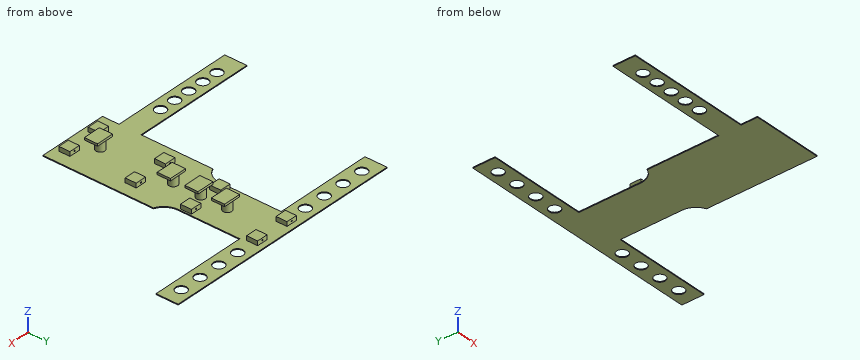
Autodesk Fusion 360 part; units mm, degrees
sketch "Sketch2" plane through (0, 0, 0) normal (0, 0, 1) x (1, 0, 0)
  circle A0 centre (0, 0) radius 11.5
  line L0 (0, 0) -> (0, -11.5)
  line L1 (9.9593, -5.75) -> (-9.9593, -5.75)
  line L2 (9.9593, -5.75) -> (-9.9593, -5.75)
  arc A1 (-9.9593, -5.75) -> (9.9593, -5.75) centre (0, 0) ccw
  dimension "d6" = 23
sketch "Sketch3" plane through (0, 0, 0) normal (0, 0, 1) x (1, 0, 0)
  line L0 (0, -37.5) -> (0, -12.5)
  line L1 (0, -12.5) -> (0, -7.5)
  line L2 (0, -7.5) -> (0, 7.5)
  line L3 (0, 7.5) -> (0, 12.5)
  line L4 (0, 12.5) -> (0, 32.5)
  line L5 (0, 32.5) -> (0, 57.5)
  line L6 (0, 57.5) -> (48, 57.5)
  line L7 (48, 57.5) -> (48, 47.5)
  line L8 (48, 47.5) -> (0, 47.5)
  line L9 (0, 47.5) -> (-48, 47.5)
  line L10 (-48, 57.5) -> (0, 57.5)
  line L11 (0, 32.5) -> (-47.7177, 32.5)
  line L12 (-24, -25) -> (-72, -25)
  line L13 (-72, -25) -> (-72, -20)
  line L14 (-72, -20) -> (-24, -20)
  line L15 (-24, -20) -> (-24, -30)
  line L16 (-24, -30) -> (-72, -30)
  line L17 (-72, -30) -> (-72, -20)
  line L18 (15.8003, -25) -> (15.8003, -28)
  line L19 (-72, -30) -> (-62, -30) construction
  line L20 (-62, -30) -> (-62, -11.1593) construction
  line L21 (-62, -30) -> (-47, -30) construction
  line L22 (-47, -30) -> (-32, -30) construction
  line L23 (-47, -30) -> (-47, -8.6093) construction
  line L24 (-32, -30) -> (-32, -9.4061) construction
  circle A0 centre (-62, -25) radius 2.5
  circle A1 centre (-47, -25) radius 2.5
  circle A2 centre (-32, -25) radius 2.5
  line L25 (-11, 22.5) -> (-11, 25.5)
  line L26 (-11, 19.5) -> (-11, 22.5)
  line L27 (12, 22.5) -> (11, 22.5)
  line L28 (11, 22.5) -> (11, 25.5)
  line L29 (11, 19.5) -> (11, 22.5)
  line L30 (48, 52.5) -> (38, 52.5) construction
  circle A3 centre (-38, 52.5) radius 2.5
  circle A4 centre (38, 52.5) radius 2.5
  line L31 (-38, 52.5) -> (-28, 52.5)
  line L32 (38, 52.5) -> (28, 52.5)
  circle A5 centre (28, 52.5) radius 2.5
  circle A6 centre (-28, 52.5) radius 2.5
  line L33 (-15.8, -12.5) -> (-15.8, 12.5)
  line L34 (11, 25.5) -> (11, 47.5)
  line L35 (-11, 25.5) -> (-11, 47.5)
  line L36 (-15.8, -12.5) -> (-15.8, -37.5)
  line L37 (15.8, 10) -> (15.8003, -22)
  line L38 (-24, -20) -> (-15.8, -20)
  line L39 (-24, -30) -> (-15.8, -30)
  line L40 (-15.8, -37.5) -> (15.8003, -37.5)
  line L41 (15.8003, -22) -> (15.8003, -37.5)
  circle A7 centre (0, -25) radius 2
  line L42 (-2, -25) -> (-3, -25)
  line L43 (-3, -25) -> (-3, -22)
  line L44 (-3, -22) -> (5, -22)
  line L45 (5, -22) -> (5, -28)
  line L46 (5, -28) -> (-3, -28)
  line L47 (-3, -28) -> (-3, -25)
  line L48 (-34.5, -25) -> (-39.5, -25)
  line L49 (-49.5, -25) -> (-54.5, -25)
  circle A8 centre (-39.5, -25) radius 2.5
  circle A9 centre (-54.5, -25) radius 2.5
  line L50 (-15.8, 12.5) -> (15.8, 12.5003)
  line L51 (15.8, 12.5003) -> (15.8, 10)
  arc A10 (-15.8, 12.5) -> (-11, 19.5) centre (-18.5042, 19.5) ccw
  arc A11 (11, 19.5) -> (15.8, 12.5003) centre (18.5037, 19.5) ccw
  circle A12 centre (23, 52.5) radius 2.5 construction
  circle A13 centre (18, 52.5) radius 2.5
  circle A14 centre (-23, 52.5) radius 2.5 construction
  circle A15 centre (-18, 52.5) radius 2.5
  circle A16 centre (43, 52.5) radius 2.5 construction
  circle A17 centre (48, 52.5) radius 2.5
  circle A18 centre (-48, 52.5) radius 2.5
  circle A19 centre (0, 32.5) radius 2
  circle A20 centre (0, 20.5) radius 2
  circle A21 centre (0, 8) radius 2
  line L52 (-2, 8) -> (-3, 8)
  line L53 (-3, 8) -> (-3, 11)
  line L54 (-3, 11) -> (5, 11)
  line L55 (5, 11) -> (5, 5)
  line L56 (5, 5) -> (-3, 5)
  line L57 (-3, 8) -> (-3, 5)
  line L58 (-2, 20.5) -> (-3, 20.5)
  line L59 (-3, 20.5) -> (-3, 23.5)
  line L60 (-3, 23.5) -> (5, 23.5)
  line L61 (5, 23.5) -> (5, 17.5)
  line L62 (5, 17.5) -> (-3, 17.5)
  line L63 (-3, 17.5) -> (-3, 20.5)
  line L64 (-2, 32.5) -> (-3, 32.5)
  line L65 (-3, 32.5) -> (-3, 35.5)
  line L66 (-3, 35.5) -> (5, 35.5)
  line L67 (5, 35.5) -> (5, 29.5)
  line L68 (5, 29.5) -> (-3, 29.5)
  line L69 (-3, 29.5) -> (-3, 32.5)
  line L70 (55.5, 57.5) -> (55.5, 47.5)
  line L71 (48, 47.5) -> (55.5, 47.5)
  line L72 (55.5, 57.5) -> (48, 57.5)
  line L73 (-55.5, 52.5) -> (-55.5, 57.5)
  line L74 (-55.5, 57.5) -> (-48, 57.5)
  line L75 (-48, 47.5) -> (-55.5, 47.5)
  line L76 (-55.5, 47.5) -> (-55.5, 52.5)
  line L77 (15.8003, -37.5) -> (7.8003, -37.5)
  line L78 (7.8003, -37.5) -> (7.8003, 57.5) construction
  line L79 (-15.8, -37.5) -> (-7.8, -37.5) construction
  line L80 (-7.8, -37.5) -> (-7.8, 57.5) construction
  line L81 (7.8003, -37.5) -> (7.8003, -32.5) construction
  line L82 (-7.8, -37.5) -> (-7.8, -32.5) construction
  line L83 (10.3003, -30) -> (5.3003, -30)
  line L84 (5.3003, -30) -> (5.3003, -35)
  line L85 (5.3003, -35) -> (10.3003, -35)
  line L86 (10.3003, -35) -> (10.3003, -30)
  line L87 (10.3003, -30) -> (5.3003, -35) construction
  line L88 (5.3003, -30) -> (10.3003, -35) construction
  line L89 (-5.3, -30) -> (-10.3, -30)
  line L90 (-10.3, -30) -> (-10.3, -35)
  line L91 (-10.3, -35) -> (-5.3, -35)
  line L92 (-5.3, -35) -> (-5.3, -30)
  line L93 (-5.3, -30) -> (-10.3, -35) construction
  line L94 (-10.3, -30) -> (-5.3, -35) construction
  line L95 (0, -37.5) -> (0, -2.5) construction
  line L96 (0, -2.5) -> (29.2324, -2.4997) construction
  line L97 (0, -2.5) -> (-32.3166, -2.4998) construction
  line L98 (-5.3, 0) -> (-10.3, 0)
  line L99 (-10.3, 0) -> (-10.3, -5)
  line L100 (-10.3, -5) -> (-5.3, -5)
  line L101 (-5.3, -5) -> (-5.3, 0)
  line L102 (-5.3, 0) -> (-10.3, -5) construction
  line L103 (-10.3, 0) -> (-5.3, -5) construction
  line L104 (10.3003, 0.0001) -> (5.3003, 0.0001)
  line L105 (5.3003, 0.0001) -> (5.3003, -4.9999)
  line L106 (5.3003, -4.9999) -> (10.3003, -4.9999)
  line L107 (10.3003, -4.9999) -> (10.3003, 0.0001)
  line L108 (10.3003, 0.0001) -> (5.3003, -4.9999) construction
  line L109 (5.3003, 0.0001) -> (10.3003, -4.9999) construction
  line L110 (0, -37.5) -> (0, 22.5) construction
  line L111 (0, 22.5) -> (29.4799, 22.5) construction
  line L112 (0, 22.5) -> (-30.0065, 22.5) construction
  line L113 (-5.3, 25) -> (-10.3, 25)
  line L114 (-10.3, 25) -> (-10.3, 20)
  line L115 (-10.3, 20) -> (-5.3, 20)
  line L116 (-5.3, 20) -> (-5.3, 25)
  line L117 (-5.3, 25) -> (-10.3, 20) construction
  line L118 (-10.3, 25) -> (-5.3, 20) construction
  line L119 (10.3003, 25) -> (5.3003, 25)
  line L120 (5.3003, 25) -> (5.3003, 20)
  line L121 (5.3003, 20) -> (10.3003, 20)
  line L122 (10.3003, 20) -> (10.3003, 25)
  line L123 (10.3003, 25) -> (5.3003, 20) construction
  line L124 (5.3003, 25) -> (10.3003, 20) construction
  line L125 (0, 47.5) -> (0, 52.5)
  line L126 (0, 52.5) -> (7.8003, 52.5) construction
  line L127 (0, 52.5) -> (-7.8, 52.5) construction
  line L128 (-5.3, 55) -> (-10.3, 55)
  line L129 (-10.3, 55) -> (-10.3, 50)
  line L130 (-10.3, 50) -> (-5.3, 50)
  line L131 (-5.3, 50) -> (-5.3, 55)
  line L132 (-5.3, 55) -> (-10.3, 50) construction
  line L133 (-10.3, 55) -> (-5.3, 50) construction
  line L134 (10.3003, 55) -> (5.3003, 55)
  line L135 (5.3003, 55) -> (5.3003, 50)
  line L136 (5.3003, 50) -> (10.3003, 50)
  line L137 (10.3003, 50) -> (10.3003, 55)
  line L138 (10.3003, 55) -> (5.3003, 50) construction
  line L139 (5.3003, 55) -> (10.3003, 50) construction
  point P0 (7.8003, -32.5)
  point P1 (-7.8, -32.5)
  point P2 (-7.8, -2.5)
  point P3 (7.8003, -2.4999)
  point P4 (-7.8, 22.5)
  point P5 (7.8003, 22.5)
  point P6 (-7.8, 52.5)
  point P7 (7.8003, 52.5)
  dimension "d9" = 25
  dimension "d10" = 5
  dimension "d11" = 15
  dimension "d12" = 5
  dimension "d13" = 20
  dimension "d14" = 25
  dimension "d15" = 48
  dimension "d16" = 10
  dimension "d17" = 48
  dimension "d18" = 10
  dimension "d20" = 48
  dimension "d22" = 5
  dimension "d23" = 10
  dimension "d28" = 10
  dimension "d29" = 15
  dimension "d30" = 15
  dimension "d31" = 5
  dimension "d32" = 5
  dimension "d33" = 5
  dimension "d40" = 3
  dimension "d43" = 1
  dimension "d44" = 3
  dimension "d49" = 10
  dimension "d53" = 5
  dimension "d55" = 5
  dimension "d57" = 10
  dimension "d58" = 10
  dimension "d59" = 5
  dimension "d60" = 5
  dimension "d75" = 4
  dimension "d76" = 1
  dimension "d77" = 3
  dimension "d78" = 8
  dimension "d79" = 6
  dimension "d80" = 5
  dimension "d81" = 5
  dimension "d82" = 5
  dimension "d83" = 5
  dimension "d84" = 5
  dimension "d85" = 5
  dimension "d86" = 5
  dimension "d87" = 5
  dimension "d88" = 5
  dimension "d89" = 5
  dimension "d91" = 5
  dimension "d94" = 4
  dimension "d97" = 4
  dimension "d99" = 4
  dimension "d100" = 1
  dimension "d101" = 3
  dimension "d102" = 8
  dimension "d103" = 6
  dimension "d104" = 1
  dimension "d105" = 3
  dimension "d106" = 8
  dimension "d107" = 6
  dimension "d108" = 1
  dimension "d109" = 3
  dimension "d110" = 8
  dimension "d111" = 6
  dimension "d122" = 8
  dimension "d123" = 8
  dimension "d124" = 5
  dimension "d125" = 5
  dimension "d126" = 5
  dimension "d127" = 5
  dimension "d128" = 5
  dimension "d129" = 5
  dimension "d130" = 35
  dimension "d131" = 5
  dimension "d132" = 5
  dimension "d133" = 5
  dimension "d134" = 5
  dimension "d135" = 60
  dimension "d136" = 5
  dimension "d137" = 5
  dimension "d138" = 5
  dimension "d139" = 5
  dimension "d140" = 5
  dimension "d141" = 5
  dimension "d142" = 5
  dimension "d143" = 5
  dimension "d144" = 5
extrude "Extrude8" add sketch "Sketch3" along normal blind 6.4 contours L0 A7 L42 L46 L47 | L0 A7 L44 L45 L46 | L0 A7 | L0 A7 | L0 A7 L42 L43 L44 | L2 A21 L52 L56 L57 | L2 L3 A21 L54 L55 L56 | L3 A21 L52 L53 L54 | L4 A20 L58 L62 L63 | L4 A20 L60 L61 L62 | L2 L3 A21 | L2 L3 A21 | L4 A20 | L4 A20 | L4 A20 L58 L59 L60 | L5 L11 A19 L64 L65 L66 | L4 L11 A19 L64 L68 L69 | L4 L5 A19 L66 L67 L68 | L5 L11 A19 | L4 L11 A19 | L4 L5 A19 makes body 1 at (-0.3333, 11, 2.1333) makes body 2 at (-0.3333, 23.5, 2.1333) makes body 3 at (-0.3333, -22, 2.1333) makes body 4 at (-0.3333, 35.5, 2.1333)
extrude "Extrude9" add sketch "Sketch3" along normal blind 0.4 contours L0 L1 L2 L3 L33 L36 L40 L43 L44 L46 L47 L50 L53 L54 L56 L57 | L0 L1 L2 L3 L18 L37 L40 L41 L44 L45 L46 L50 L51 L54 L55 L56 L77 | L15 L36 L38 L39 | L12 L15 L16 L17 A0 A1 A2 L48 L49 A8 A9 | L12 L13 L14 L15 L17 A0 A1 A2 L48 L49 A8 A9 | L4 L11 L25 L26 L35 L50 A10 L59 L60 L62 L63 L68 L69 | L4 L5 L8 L28 L29 L34 L50 A11 L60 L61 L62 L66 L67 L68 | L5 L9 L11 L35 L65 L66 | L5 L9 L10 L73 L74 L75 L76 L125 | L5 L6 L7 L8 A17 L125 | L7 A17 L70 L71 L72 | L113 L114 L115 L116 | L119 L120 L121 L122 | L128 L129 L130 L131 | L134 L135 L136 L137 bodies 1 2 3 4
extrude "Extrude10" cut sketch "Sketch3" along normal blind 5.4 contours L0 A7 L42 L46 L47 | L0 A7 L44 L45 L46 | L0 A7 L42 L43 L44 | L2 A21 L52 L56 L57 | L2 L3 A21 L54 L55 L56 | L3 A21 L52 L53 L54 | L4 A20 L58 L62 L63 | L4 A20 L60 L61 L62 | L4 A20 L58 L59 L60 | L5 L11 A19 L64 L65 L66 | L4 L11 A19 L64 L68 L69 | L4 L5 A19 L66 L67 L68 bodies 1 makes body 5 at (1.9901, 32.6991, 3.6) makes body 6 at (1.9901, 20.6991, 1.8) makes body 7 at (1.9901, 7.8009, 3.6) makes body 8 at (1.9901, -24.8009, 1.8)
extrude "Extrude11" add sketch "Sketch3" along normal blind 0.4 contours L0 A7 L42 L46 L47 | L0 A7 L44 L45 L46 | L0 A7 L42 L43 L44 | L2 A21 L52 L56 L57 | L2 L3 A21 L54 L55 L56 | L3 A21 L52 L53 L54 | L4 A20 L58 L62 L63 | L4 A20 L60 L61 L62 | L4 A20 L58 L59 L60 | L5 L11 A19 L64 L65 L66 | L4 L11 A19 L64 L68 L69 | L4 L5 A19 L66 L67 L68 bodies 1 5 6 7 8
extrude "Extrude12" add sketch "Sketch3" along normal blind 3.4 contours L83 L84 L85 L86 | L89 L90 L91 L92 | L98 L99 L100 L101 | L104 L105 L106 L107 | L113 L114 L115 L116 | L119 L120 L121 L122 | L128 L129 L130 L131 | L134 L135 L136 L137 bodies 1
extrude "Extrude13" cut 8 faces at (-8.6333, 53.3333, 3.4) (6.967, 53.3333, 3.4) (-8.6333, 23.3333, 3.4) (6.967, 23.3333, 3.4) (-8.6333, -1.6666, 3.4) (6.967, -1.6666, 3.4) (6.967, -33.3333, 3.4) (-8.6333, -33.3333, 3.4) along direction (0, 0, -1) blind 1 on bodies 1 bodies 1
hole "Hole1" at (7.8003, -35, 1.4) direction (0, 1, 0) diameter 0.6 end through all bodies 1 1
hole "Hole2" at (-7.8, -35, 1.4) direction (0, 1, 0) diameter 0.6 end through all bodies 1 1
CAD build for the part. Positions are in the model's coordinates, mm. Round coordinates to 2 decimals unless told otherwise and drop trailing zeros. Order: outer loops, then holes, each group sorted by start corner. A loop starts at its lowest first (then second) coordinate and runs counter-clockwise, first axis right, second up. Notation, with made-up numbers: (-29, -26) -> (-17, -26) arc R24 ccw to (-17, 10) -> close; hole circle Ø4 at (70, 18). An arc over 180 degrees is marked (long way). Write item = value, one per line.
(1) Cut at B-B (x = 28). Write the cut outline in (y, z), plus the area to 3 significant figures.
Answers follow:
outline = (47.5, 0) -> (50, 0) -> (50, 0.4) -> (47.5, 0.4) -> close; (55, 0) -> (57.5, 0) -> (57.5, 0.4) -> (55, 0.4) -> close
area = 2.00 mm²
(2) Cut at A-A (x = -28). Write the cut outline in (y, z).
Answers follow:
outline = (-30, 0) -> (-20, 0) -> (-20, 0.4) -> (-30, 0.4) -> close; (47.5, 0) -> (50, 0) -> (50, 0.4) -> (47.5, 0.4) -> close; (55, 0) -> (57.5, 0) -> (57.5, 0.4) -> (55, 0.4) -> close
(3) Drill centre lines: L1, parallel to Y at x = -28, z = 0.3; L2, parallel to Y at x = -47, z = 0.2; L3, parallel to Y at x = 48, z = 0.15. Where is each one in solid material? Low to high.
Answers follow:
L1 = -30 to -20, 47.5 to 50, 55 to 57.5
L2 = -30 to -27.5, -22.5 to -20, 47.5 to 50.21, 54.79 to 57.5
L3 = 47.5 to 50, 55 to 57.5
(4) Cut at C-C (y = -25). State how many separate pieces and enclosed holes the cut face has, plus the area to 3 significant figures.
Answers follow:
separate_pieces = 6
enclosed_holes = 0
area = 53.1 mm²
(5) Flat gauge pins, fed straight in: P1, Ø4, axis at x = 8, y = -2.5, coming from the +Z side; P2, Ø1, axis at y = 22, z = 1, coming from the -X side; P3, Ø1, axis at x = -1, y = 46.5, coming from the +Z side; P4, Ø2, axis at x = 8.5, z = 1, coming from the +Y side. Where does each tip first touch, or does it go through?
Answers follow:
P1 = 2.4
P2 = -10.3
P3 = 0.4
P4 = 57.5
(6) Cut at D-D (z = 3.75). Write the cut outline in (x, y).
Answers follow:
outline = circle Ø4 at (0, -25); circle Ø4 at (0, 8); circle Ø4 at (0, 20.5); circle Ø4 at (0, 32.5)
